Solid Edge part; units mm, degrees
sketch "Sketch1" plane through (0, 0, 0) normal (0, -1, 0) x (1, 0, 0)
  line L0 (42.8, 115.9) -> (42.8, 66.8363)
  line L1 (42.8, 66.8363) -> (55, 54.6363)
  line L2 (55, 54.6363) -> (55, 0)
  line L3 (55, 0) -> (63, 0)
  line L4 (63, 0) -> (67, 0)
  line L5 (67, 0) -> (67, 8)
  line L6 (67, 8) -> (63, 12)
  line L7 (63, 12) -> (63, 57.95)
  line L8 (63, 57.95) -> (50.8, 70.15)
  line L9 (50.8, 115.9) -> (50.8, 70.15)
  line L10 (42.8, 115.9) -> (50.8, 115.9)
revolve "RevolvedProtrusion1" add sketch "Sketch1" angle 360 about axis through (0, 0, 0) along (0, 0, 1)
chamfer "Chamfer1" distance 3 angle 45 1 edges at (-50.8, 0, 115.9)
Here's how the part is built. I have some questions about the finished solid (model axes, mm). A direction names the side the tool comes from. Coordinates: 2 decimals unless noted, no trailing zeros. Write each loop counter-clockwise with the first axis right and the second up, starting at its lowest first coordinate (ties: lowest second). Pieces come first, ordered by that corner, then holes. Notation, with made-up numbers: (35, 7) - (46, 7) arc R9 cw to (46, 24) - close; hole circle Ø7 at (7, 6.25). An arc over 180 degrees is marked (long way). One line per item, written item: value.
1) We'd pull the mould along X, two halves only. Please class faces 3 (the cylindrical face through (-8.201, 62.464, 35.297)), 4 (the flat face through (-36, -25, 115.9)), 5 (the cylindrical face through (-11.923, 53.692, 26.936)): pulls with the +X half, pulls with the -X half, needs draft (parallel to the pull), parting line crosses it, or undercut.
Model answer:
face 3: parting line crosses it
face 4: needs draft
face 5: undercut
2) Suppose I cut it at A-A on y = 0. Write out the boundary of the cut face in (x, z), and give its area (3 significant figures).
Model answer:
outline: (-67, 0) - (-55, 0) - (-55, 54.64) - (-42.8, 66.84) - (-42.8, 115.9) - (-47.8, 115.9) - (-50.8, 112.9) - (-50.8, 70.15) - (-63, 57.95) - (-63, 12) - (-67, 8) - close; (42.8, 66.84) - (55, 54.64) - (55, 0) - (67, 0) - (67, 8) - (63, 12) - (63, 57.95) - (50.8, 70.15) - (50.8, 112.9) - (47.8, 115.9) - (42.8, 115.9) - close
area: 2,010 mm²
3) On a 3-axis mill with a long thin cutter (end or side, diameter ignored), from which of +Z, -Z, +X, -X, +Y, -Y can I reach the whole of each face in a straight line? I mean faces 1 (the cylindrical face through (-9.28, 41.78, 91.02)), 2 (the cylindrical face through (-11.012, 49.592, 91.226)). Say none if no direction works.
Model answer:
face 1: +Z, -Z
face 2: +Z
4) I need wall thicknesses on line 1 along Y through (x, z) = (0, 20.5); line 2 along Y through (x, z) = (25.5, 63); line 3 along X through (y, z) = (34.5, 103). Which ranges of each line are inside material? Lowest first, please.
Model answer:
line 1: y = -63 to -55, 55 to 63
line 2: y = -52.04 to -39.05, 39.05 to 52.04
line 3: x = -37.29 to -25.33, 25.33 to 37.29
5) I'm going to push flat-ended pins straight in: P1, Ø1.5, axis at x = 24, z = 104, coming from the +Y side; P2, Ø2, axis at y = -0.5, z = 51.5, coming from the -X side; P3, Ø1.5, axis at x = 41, y = 33.5, coming from the -Z side. Where does each tip first touch, or does it pass through?
Model answer:
P1: stops at y = 45.17
P2: stops at x = -63
P3: stops at z = 55.94
6) Suppose I cut it at D-D on z = 43. Write out the boundary of the cut face in (x, y), and give its area (3 significant figures).
Model answer:
outline: circle Ø126 at (0, 0); hole circle Ø110 at (0, 0)
area: 2,970 mm²
7) Suppose I cut it at C-C on z = 82. Write out the boundary of the cut face in (x, y).
Model answer:
outline: circle Ø101.6 at (0, 0); hole circle Ø85.6 at (0, 0)
